Geometry: final body of the model. Coordinates: model frame, mm. Face numbers are marked on the shaded views. A direction names the side the tool comes from. Give positions to 0.01 mm unless a question says otherwise; leave off trailing zeros. Loops run counter-clockwise (first coordinate to the right, second up) from the corner with the lowest first, then second, coordinate; pieces in that order, holes last.
Solid Edge part; units mm, degrees
sketch "Sketch1" plane through (0, 0, 0) normal (0, 0, 1) x (1, 0, 0)
  circle A0 centre (0, 0) radius 1.425
extrude "Protrusion1" add sketch "Sketch1" against normal blind 10
sketch "Sketch2" plane through (0, 0, 0) normal (0, 0, 1) x (1, 0, 0)
  circle A0 centre (0, 0) radius 2.75
extrude "ExtrudedProtrusion_2" add sketch "Sketch2" along normal blind 2
sketch "Sketch3" plane through (0, 0, 2) normal (0, 0, 1) x (1, 0, 0)
  line L0 (3.6964, 0.4) -> (-3.6964, 0.4)
  line L1 (-3.6964, 0.4) -> (-3.6964, -0.4)
  line L2 (-3.6964, -0.4) -> (3.6964, -0.4)
  line L3 (3.6964, -0.4) -> (3.6964, 0.4)
extrude "ExtrudedCutout_1" cut sketch "Sketch3" against normal blind 0.5
properties material "Graphite"
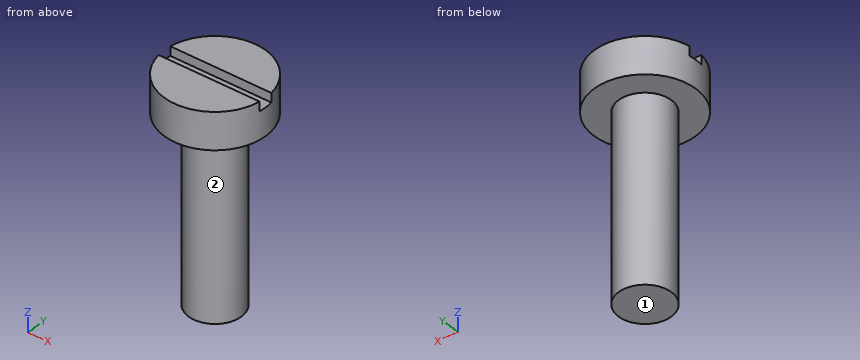
Item 1: Pin query (flat end, axial travel): pin 1 (1 mm diameter, centred on x = -0.5, y = 0, fed in from +Z); pin 2 (1.5 mm diameter, centred on y = 2, z = -7, fed in from -X). Return the tip coordinate at first contact, or that it passes through.
Values follow:
pin 1: stops at z = 2
pin 2: stops at x = -0.68
Item 2: Section query B-B on y = 0. Return loops of the section in (x, z) (3 decimals).
Values follow:
outline: (-2.75, 0) - (-1.425, 0) - (-1.425, -10) - (1.425, -10) - (1.425, 0) - (2.75, 0) - (2.75, 1.5) - (-2.75, 1.5) - close
Item 3: Ray query, probe 1 along Z at (x, y) = (0.75, 2.55); probe 2 along Y at (x, z) = (0.1, -8.25); probe 3 along Z at (x, y) = (0.6, -0.15). Return the intervals inside material, ascending.
Values follow:
probe 1: z = 0 to 2
probe 2: y = -1.42 to 1.42
probe 3: z = -10 to 1.5
Item 4: Section query D-D on y = -1.05. Return loops of the section in (x, z).
Values follow:
outline: (-2.54, 0) - (-0.96, 0) - (-0.96, -10) - (0.96, -10) - (0.96, 0) - (2.54, 0) - (2.54, 2) - (-2.54, 2) - close
Item 5: Section query C-C on z = 0.75. Return loops of the section in (x, y).
Values follow:
outline: circle Ø5.5 at (0, 0)
Item 6: Section query A-A on x = 0. Return loops of the section in (y, z) (3 decimals).
Values follow:
outline: (-2.75, 0) - (-1.425, 0) - (-1.425, -10) - (1.425, -10) - (1.425, 0) - (2.75, 0) - (2.75, 2) - (0.4, 2) - (0.4, 1.5) - (-0.4, 1.5) - (-0.4, 2) - (-2.75, 2) - close
Item 7: Set-up query: the marked faces 1 and 2. Return all of +Z, -Z, +X, -X, +Y, -Y with unobstructed straight access to the full face (end or side cutting, diameter ignored); none if empty.
Values follow:
face 1: -Z, +X, -X, +Y, -Y
face 2: -Z
